from build123d import *

# Parameters (mm, degrees)
F1_DEPTH = 50.8
F2_R     = 1.98374
F3_R     = 3.69316
F4_R     = 1.8288
F5_DEPTH = 1.70942
F6_R     = 1.8288
F7_DEPTH = 1.70942
F8_R     = 4.7625


with BuildPart() as f1:
    # F0 (on Top) → F1 (new body)
    with BuildSketch(Plane.XY):
        Polygon((1.70942, 25.4), (0, 25.4), (0, 0), (-25.4, 0), (-25.4, -1.70942), (1.70942, -1.70942), align=None)
    extrude(amount=F1_DEPTH)

    # F2
    f2_edges = [f1.edges().sort_by_distance(p)[0] for p in [
        (0, 0, 25.4),
    ]]
    fillet(f2_edges, radius=F2_R)

    # F3
    f3_edges = [f1.edges().sort_by_distance(p)[0] for p in [
        (1.70942, -1.70942, 25.4),
    ]]
    fillet(f3_edges, radius=F3_R)

    # F4 (on face) → F5 (cut, through all)
    with BuildSketch(Plane(origin=(0, 0, 0), x_dir=(0, -1, 0), z_dir=(-1, 0, 0))):
        with Locations((-20.6375, 46.0375)):
            Circle(F4_R)
        with Locations((-20.6375, 4.7625)):
            Circle(F4_R)
    extrude(amount=-F5_DEPTH, mode=Mode.SUBTRACT)

    # F6 (on face) → F7 (cut, through all)
    with BuildSketch(Plane(origin=(0, 0, 0), x_dir=(-1, 0, 0), z_dir=(0, 1, 0))):
        with Locations((20.6375, 46.0375)):
            Circle(F6_R)
        with Locations((20.6375, 4.7625)):
            Circle(F6_R)
    extrude(amount=-F7_DEPTH, mode=Mode.SUBTRACT)

    # F8
    f8_edges = [f1.edges().sort_by_distance(p)[0] for p in [
        (0.85471, 25.4, 50.8),
        (-25.4, -0.85471, 50.8),
        (-25.4, -0.85471, 0),
        (0.85471, 25.4, 0),
    ]]
    fillet(f8_edges, radius=F8_R)


solid = f1.part
Geometry check sheet. Reference: the model listing, model coordinates, mm. A direction names the side the tool comes from. Coordinates: 2 decimals unless noted, no trailing zeros. Order: outer loops, then holes, each group sorted by start corner. A loop starts at its lowest first (then second) coordinate and runs counter-clockwise, first axis right, second up. Notation, with made-up numbers: (68.5, 29.5) -> (93.5, 29.5) arc R19 ccw to (93.5, 41.5) -> close; hole circle Ø6 at (84.5, -18.5). An arc over 180 degrees is marked (long way). Use a Markdown table: item, result. Add a question column.
1. Go/stop test with a flat-tipped pin: pin 1 Ø6 at (y, z) = (20.64, 46.04) entering from -X. Record where the tip stops, or that it passes through.
2. Material ranges on L1, parallel to X at y = 7, z = 7; L2, parallel to Y at x = -18.25, z = 33; L3, parallel to X at y = 1, z = 4.5, recorded low to high.
3. Cross-section at B-B (z = 23). Enter the section's corners in (x, y).
4. Cross-section at A-A (x = -21.5). Enter the section's corners in (y, z).
5. Mould release check, pull along Z, two halves, no side actions. Record for faces 3 (the face through (-18.81, -0.84, 46.12)), 4 (the face through (-4.6, -0.4, 50.8)), 5 (the face through (0.843, 18.893, 46.587)), 6 (the face through (-25.4, -1, 25)): pulls with the +Z half, pulls with the -Z half, needs draft (parallel to the pull), parting line crosses it, or undercut.
6. Cross-section at D-D (y = 17). Enter the section's corners in (x, z).
7. Cross-section at C-C (z = 45). Enter the section's corners in (x, y).
8. Set-up check for faces 1 (the face through (0, 14, 25)), 2 (the face through (0.84, 24.04, 49.37)): record each of +Z, -Z, +X, -X, +Y, -Y from which the full face is reachable in a straight line by a thin tool's end or side.
Filled sheet:
| question | item | result |
|---|---|---|
| 1 | pin 1 | x = 0 |
| 2 | L1 | 0 to 1.71 |
| 2 | L2 | -1.71 to 0 |
| 2 | L3 | -0.26 to 1.58 |
| 3 | outline | (-25.4, -1.71) -> (-1.98, -1.71) arc R3.69 ccw to (1.71, 1.98) -> (1.71, 25.4) -> (0, 25.4) -> (0, 1.98) arc R1.98 cw to (-1.98, 0) -> (-25.4, 0) -> close |
| 4 | outline | (-1.71, 0.08) -> (0, 0.08) -> (0, 3.15) -> (-1.71, 3.15) -> close; (-1.71, 6.38) -> (0, 6.38) -> (0, 44.42) -> (-1.71, 44.42) -> close; (-1.71, 47.65) -> (0, 47.65) -> (0, 50.72) -> (-1.71, 50.72) -> close |
| 5 | face 3 | undercut |
| 5 | face 4 | pulls with the +Z half |
| 5 | face 5 | undercut |
| 5 | face 6 | needs draft |
| 6 | outline | (0, 0) -> (1.71, 0) -> (1.71, 50.8) -> (0, 50.8) -> close |
| 7 | outline | (-25.4, -1.71) -> (-22.14, -1.71) -> (-22.14, 0) -> (-25.4, 0) -> close; (-19.13, -1.71) -> (-1.98, -1.71) arc R3.69 ccw to (1.71, 1.98) -> (1.71, 19.13) -> (0, 19.13) -> (0, 1.98) arc R1.98 cw to (-1.98, 0) -> (-19.13, 0) -> close; (0, 22.14) -> (1.71, 22.14) -> (1.71, 25.4) -> (0, 25.4) -> close |
| 8 | face 1 | +Z, -Z, -X, +Y |
| 8 | face 2 | +Z, +X, -X, +Y |
